Print and shaded views of the part. All mm, measured from the part's lowest x, y and z. A direction names the side the tool comes from. Round coordinates to 2 decimals unless told otherwise and drop trailing zeros. Write each loop counter-clockwise with the first axis right and the second up, starting at its lowest first coordinate (ties: lowest second). Pieces come first, ordered by that corner, then holes.
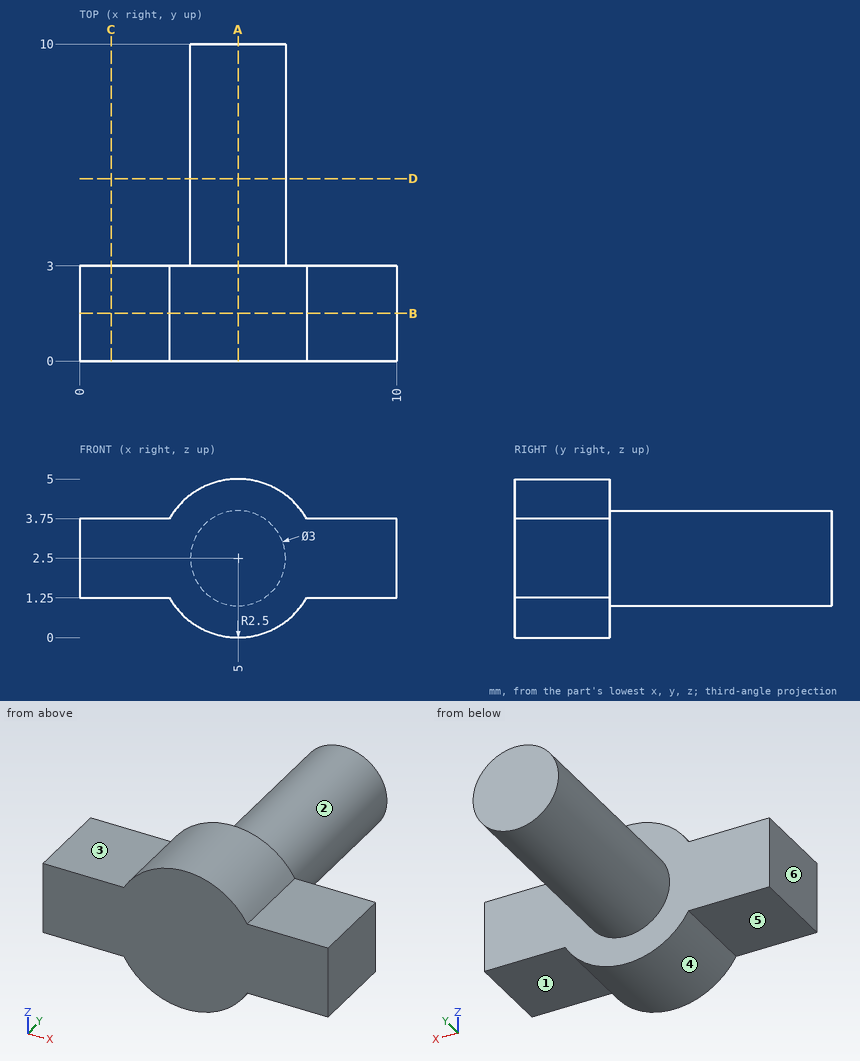
1) Mould opens along X. For the marked faces 4, 5 and 6 say: released by +X, released by -X, zero draft, split by the parting line, or undercut.
Results:
face 4: split by the parting line
face 5: zero draft
face 6: released by -X
2) Slice it at A-A (x = 5). Write the cut outline in (y, z), plus the area to 3 significant figures.
Results:
outline: (0, 0) - (3, 0) - (3, 1) - (10, 1) - (10, 4) - (3, 4) - (3, 5) - (0, 5) - close
area: 36.0 mm2
3) Slice it at D-D (y = 5.75). Write the cut outline in (x, z).
Results:
outline: circle Ø3 at (5, 2.5)
4) Pin check, flat tips, straight feed: pin 1 Ø2 at (y, z) = (6.5, 4) entering from +X; pin 2 Ø2.5 at (x, y) = (1, 1.5) entering from -Z; pin 3 Ø6 at (x, y) = (3, 8) entering from -Z. Stop position of each tip, or through.
Results:
pin 1: stops at x = 6.41
pin 2: stops at z = 1.25
pin 3: stops at z = 1
5) Which spindle directions (+Z, -Z, +X, -X, +Y, -Y) get a long thin tool onto all of the face, cutting with end or side? Do the marked faces 1, 2 and 3. Say none if no direction does.
Results:
face 1: -Z, +X, +Y, -Y
face 2: +Y
face 3: +Z, -X, +Y, -Y
6) Slice it at C-C (x = 1). Write the cut outline in (y, z), plus the area to 3 significant figures.
Results:
outline: (0, 1.25) - (3, 1.25) - (3, 3.75) - (0, 3.75) - close
area: 7.50 mm2
7) Wall check: L1, parallel to Z at x = 2.75, y = 1; L2, parallel to Y at x = 5.5, z = 0.5; L3, parallel to X at y = 5.5, z = 2.55. Give the ranges that are in metal, low to high.
Results:
L1: z = 1.25 to 3.75
L2: y = 0 to 3
L3: x = 3.5 to 6.5
8) Slice it at B-B (y = 1.5). Write the cut outline in (x, z).
Results:
outline: (0, 1.25) - (2.83, 1.25) arc R2.5 ccw to (7.17, 1.25) - (10, 1.25) - (10, 3.75) - (7.17, 3.75) arc R2.5 ccw to (2.83, 3.75) - (0, 3.75) - close
